Source: CAD feature listing. Evaluate the final solid. Frame: model axes, mm. Face numbers are marked on the shaded views. A direction names the side the tool comes from. Give positions to 0.01 mm unless a question says otherwise; leave off trailing zeros. Order: outer loops, then holes, each group sorted by start corner. A loop starts at its lowest first (then second) coordinate and runs counter-clockwise, first axis right, second up. Notation, with made-up numbers: (7.25, 28.25) -> (31.25, 28.25) arc R28 cw to (31.25, 62.25) -> close; hole circle Ø8 at (-12.75, -17.75). An arc over 180 degrees is marked (long way). Answer in a Markdown table with one row per item.
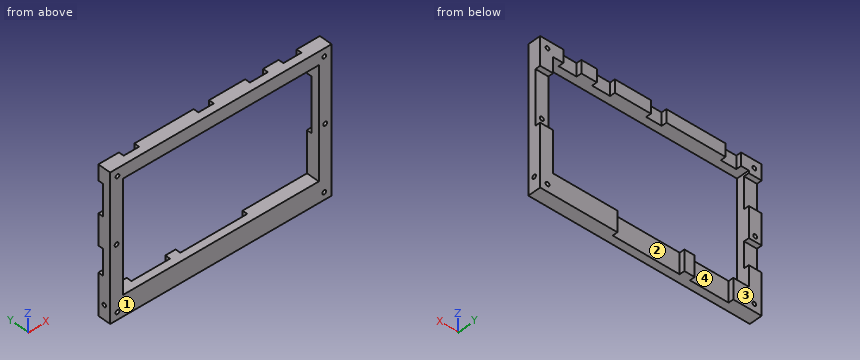
```python
from build123d import *

# Parameters (mm, degrees)
SKETCH_1_W          = 86
SKETCH_1_H          = 174
SKETCH_1_W_2        = 50
SKETCH_1_H_2        = 25
SKETCH_1_H_3        = 55
SKETCH_1_W_3        = 76
SKETCH_1_H_4        = 43
EXTRUDE_1_DEPTH     = 5
SKETCH_4_W          = 68.7
SKETCH_4_H          = 115
SKETCH_4_W_2        = 64.7
SKETCH_4_H_2        = 37
SKETCH_4_H_3        = 70
EXTRUDE_2_DEPTH     = 10
SKETCH_5_R          = 0.75
CUT_EXTRUDE_1_DEPTH = 122.783619588
SKETCH_7_W          = 15
SKETCH_7_H          = 8
SKETCH_7_W_2        = 26
SKETCH_7_W_3        = 5
SKETCH_7_H_2        = 10
SKETCH_7_H_3        = 12.119700025
SKETCH_7_W_4        = 6
SKETCH_7_H_4        = 5
SKETCH_7_W_5        = 7
SKETCH_7_H_5        = 21
CUT_EXTRUDE_2_DEPTH = 2
SKETCH_8_R          = 0.75
CUT_EXTRUDE_3_DEPTH = 2
CUT_EXTRUDE_START   = -84
SKETCH_8_3_R        = 0.75
CUT_EXTRUDE_4_DEPTH = 2
SKETCH_9_W          = 86
SKETCH_9_H          = 118
SKETCH_9_R          = 0.75
SKETCH_9_W_2        = 50
SKETCH_9_H_2        = 55
SKETCH_9_H_3        = 25
CUT_EXTRUDE_5_DEPTH = 123.295748086


with BuildPart() as part:
    # 草图1 → 凸台-拉伸1 (new body)
    with BuildSketch(Plane(origin=(0, 0, 0), x_dir=(1, 0, 0), z_dir=(0, 1, 0))):
        with Locations((0, -26.5)):
            Rectangle(SKETCH_1_W, SKETCH_1_H)
        with Locations((0, -38)):
            Rectangle(SKETCH_1_W_2, SKETCH_1_H_2, mode=Mode.SUBTRACT)
        with Locations((0, 23)):
            Rectangle(SKETCH_1_W_2, SKETCH_1_H_3, mode=Mode.SUBTRACT)
        with Locations((0, -87)):
            Rectangle(SKETCH_1_W_3, SKETCH_1_H_4, mode=Mode.SUBTRACT)
    extrude(amount=EXTRUDE_1_DEPTH)

    # 草图4 → 凸台-拉伸2 (add)
    with BuildSketch(Plane(origin=(0, 5, 0), x_dir=(1, 0, 0), z_dir=(0, 1, 0))):
        Rectangle(SKETCH_4_W, SKETCH_4_H)
        with Locations((0, -37)):
            Rectangle(SKETCH_4_W_2, SKETCH_4_H_2, mode=Mode.SUBTRACT)
        with Locations((0, 20.5)):
            Rectangle(SKETCH_4_W_2, SKETCH_4_H_3, mode=Mode.SUBTRACT)
    extrude(amount=EXTRUDE_2_DEPTH)

    # 草图5 → 切除-拉伸1 (cut, through all)
    with BuildSketch(Plane(origin=(0, 5, 0), x_dir=(1, 0, 0), z_dir=(0, 1, 0))):
        with Locations(Location((-39, 20.5, 0), (0, 0, 270))):
            Circle(SKETCH_5_R)
        with Locations(Location((39, 20.5, 0), (0, 0, 270))):
            Circle(SKETCH_5_R)
        with Locations(Location((-39, -32.5, 0), (0, 0, 270))):
            Circle(SKETCH_5_R)
        with Locations(Location((39, -32.5, 0), (0, 0, 270))):
            Circle(SKETCH_5_R)
        with Locations(Location((-40.1427775, -60.35, 0), (0, 0, 270))):
            Circle(SKETCH_5_R)
        with Locations(Location((40.1427775, -60.35, 0), (0, 0, 270))):
            Circle(SKETCH_5_R)
        with Locations(Location((-40.1427775, -110.530299975, 0), (0, 0, 270))):
            Circle(SKETCH_5_R)
        with Locations(Location((40.1427775, -110.530299975, 0), (0, 0, 270))):
            Circle(SKETCH_5_R)
        with Locations(Location((-40.5, 57.5, 0), (0, 0, 270))):
            Circle(SKETCH_5_R)
        with Locations(Location((-40.5, -38, 0), (0, 0, 270))):
            Circle(SKETCH_5_R)
        with Locations(Location((-40.5, -85.5, 0), (0, 0, 270))):
            Circle(SKETCH_5_R)
        with Locations(Location((40.5, 57.5, 0), (0, 0, 270))):
            Circle(SKETCH_5_R)
        with Locations(Location((40.5, -38, 0), (0, 0, 270))):
            Circle(SKETCH_5_R)
        with Locations(Location((40.5, -85.5, 0), (0, 0, 270))):
            Circle(SKETCH_5_R)
        with Locations(Location((-40.5, -4.5, 0), (0, 0, 270))):
            Circle(SKETCH_5_R)
        with Locations(Location((40.5, -4.5, 0), (0, 0, 270))):
            Circle(SKETCH_5_R)
    extrude(amount=-CUT_EXTRUDE_1_DEPTH, mode=Mode.SUBTRACT)

    # 草图7 → 切除-拉伸2 (cut)
    with BuildSketch(Plane(origin=(0, 5, 0), x_dir=(1, 0, 0), z_dir=(0, 1, 0))):
        with Locations((-24.5, -61.5)):
            Rectangle(SKETCH_7_W, SKETCH_7_H)
        with Locations((0, -61.5)):
            Rectangle(SKETCH_7_W_2, SKETCH_7_H)
        with Locations((-40.5, -78.5)):
            Rectangle(SKETCH_7_W_3, SKETCH_7_H_2)
        with Locations((-40.5, -101.440149988)):
            Rectangle(SKETCH_7_W_3, SKETCH_7_H_3)
        with Locations((-32, -111)):
            Rectangle(SKETCH_7_W_4, SKETCH_7_H_4)
        with Locations((-3, -111)):
            Rectangle(SKETCH_7_W_4, SKETCH_7_H_4)
        with Locations((17.5, -111)):
            Rectangle(SKETCH_7_W_5, SKETCH_7_H_4)
        with Locations((30.5, -111)):
            Rectangle(SKETCH_7_W_5, SKETCH_7_H_4)
        with Locations((40.5, -92)):
            Rectangle(SKETCH_7_W_3, SKETCH_7_H_5)
    extrude(amount=-CUT_EXTRUDE_2_DEPTH, mode=Mode.SUBTRACT)

    # 草图8 → 切除-拉伸3 (cut)
    with BuildSketch(Plane.ZY.offset(43)):
        with Locations((8, 2.5)):
            Circle(SKETCH_8_R)
        with Locations((23, 2.5)):
            Circle(SKETCH_8_R)
        with Locations((52, 2.5)):
            Circle(SKETCH_8_R)
        with Locations((63, 2.5)):
            Circle(SKETCH_8_R)
    extrude(amount=-CUT_EXTRUDE_3_DEPTH, mode=Mode.SUBTRACT)

    # 草图8<3> → 切除-拉伸4 (cut)
    with BuildSketch(Plane.ZY.offset(43).offset(CUT_EXTRUDE_START)):
        with Locations((8, 2.5)):
            Circle(SKETCH_8_3_R)
        with Locations((23, 2.5)):
            Circle(SKETCH_8_3_R)
        with Locations((52, 2.5)):
            Circle(SKETCH_8_3_R)
        with Locations((63, 2.5)):
            Circle(SKETCH_8_3_R)
    extrude(amount=-CUT_EXTRUDE_4_DEPTH, mode=Mode.SUBTRACT)

    # 草图9 → 切除-拉伸5 (cut, through all)
    with BuildSketch(Plane(origin=(0, 0, 0), x_dir=(1, 0, 0), z_dir=(0, 1, 0))):
        with Locations((0, 1.5)):
            Rectangle(SKETCH_9_W, SKETCH_9_H)
        with Locations((-40.5, -4.5)):
            Circle(SKETCH_9_R, mode=Mode.SUBTRACT)
        with Locations((-39, 20.5)):
            Circle(SKETCH_9_R, mode=Mode.SUBTRACT)
        with Locations((-40.5, 57.5)):
            Circle(SKETCH_9_R, mode=Mode.SUBTRACT)
        with Locations((0, 23)):
            Rectangle(SKETCH_9_W_2, SKETCH_9_H_2, mode=Mode.SUBTRACT)
        with Locations((40.5, -4.5)):
            Circle(SKETCH_9_R, mode=Mode.SUBTRACT)
        with Locations((39, 20.5)):
            Circle(SKETCH_9_R, mode=Mode.SUBTRACT)
        with Locations((40.5, 57.5)):
            Circle(SKETCH_9_R, mode=Mode.SUBTRACT)
        with Locations((39, -32.5)):
            Circle(SKETCH_9_R, mode=Mode.SUBTRACT)
        with Locations((-40.5, -38)):
            Circle(SKETCH_9_R, mode=Mode.SUBTRACT)
        with Locations((-39, -32.5)):
            Circle(SKETCH_9_R, mode=Mode.SUBTRACT)
        with Locations((0, -38)):
            Rectangle(SKETCH_9_W_2, SKETCH_9_H_3, mode=Mode.SUBTRACT)
        with Locations((40.5, -38)):
            Circle(SKETCH_9_R, mode=Mode.SUBTRACT)
    extrude(amount=CUT_EXTRUDE_5_DEPTH, mode=Mode.SUBTRACT)


solid = part.part
```
(1) Access query for the marked faces 3 and 4. Directions: +Z, -Z, +X, -X, +Y, -Y. A direction counts if a zero-diameter tool reaches every point of the face in a straight line with its end or side. Return the directions, or none.
A:
| item | result |
|---|---|
| face 3 | +Z, -Z, +X, -X, +Y |
| face 4 | -Z, +Y |
(2) Section query A-A (x = 35). Return the cut outline in (y, z), plus the area to 3 significant figures.
A:
| item | result |
|---|---|
| outline | (0, 57.5) -> (5, 57.5) -> (5, 65.5) -> (0, 65.5) -> close; (0, 108.5) -> (5, 108.5) -> (5, 113.5) -> (0, 113.5) -> close |
| area | 65.0 mm^2 |
(3) Ray query, probe 1 along X at (y, z) = (2.8, 85.5); probe 2 along X at (y, z) = (3.4, 60.35); probe 3 along Z at (x, y) = (-35, 0.85). Return the intervals inside material, ascending.
A:
| item | result |
|---|---|
| probe 1 | x = -43 to -41.25, -39.75 to -38, 38 to 39.75, 41.25 to 43 |
| probe 2 | x = -43 to -40.89, -39.39 to -32, -17 to -13, 13 to 39.39, 40.89 to 43 |
| probe 3 | z = 57.5 to 65.5, 108.5 to 113.5 |
(4) Section query B-B (z = 69.5). Return the cut outline in (x, y).
A:
| item | result |
|---|---|
| outline | (-43, 0) -> (-38, 0) -> (-38, 5) -> (-43, 5) -> close; (38, 0) -> (43, 0) -> (43, 5) -> (38, 5) -> close |
(5) Pull-direction query (X, two-part tool) for the marked faces 1 and 2; classes: +X half, -X half, draft (parallel to the pull), parting line (faces both ways), or undercut.
A:
| item | result |
|---|---|
| face 1 | draft |
| face 2 | undercut |
(6) First-contact query: pin 1 Ø4 at (x, z) = (41, 91.5) entering from +Y; pin 2 Ø1.7 at (x, z) = (40.14, 60.35) entering from +Y. Flat tips, straight axial feed; report the tip coordinate or a pass-through.
A:
| item | result |
|---|---|
| pin 1 | stops at y = 3 |
| pin 2 | stops at y = 5 |
